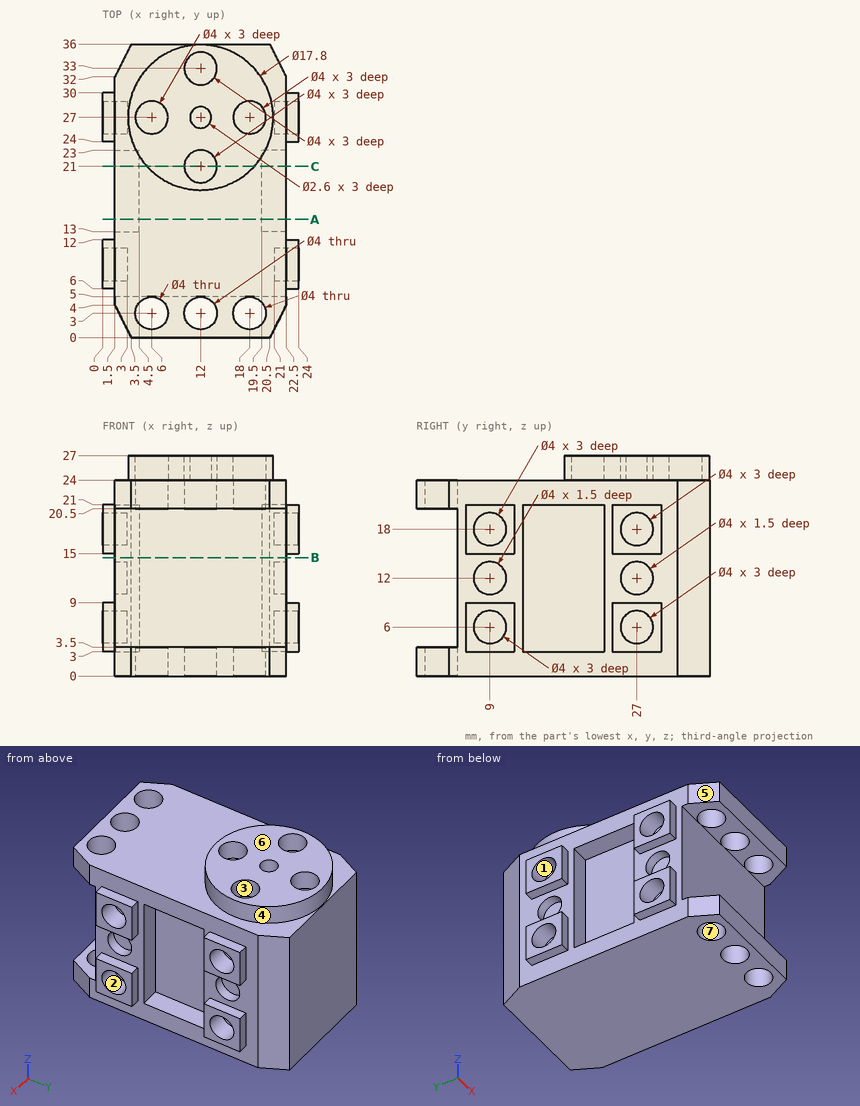
Answer from the drawing. Dimensions are ordinates in mm from the lowest x, y and z of the part. A direction names the side the tool comes from. Give positions to 0.01 mm unless a question says otherwise; leave off trailing zeros. Write each loop counter-clockwise with the first axis right and the second up, starting at its lowest first coordinate (ties: lowest second). Pieces come first, ordered by that corner, then holes.
1) Find the intervals of material crossed by L1, parallel to Y at x = 1.3, z = 6; L2, parallel to Y at x = 12, z = 2.8; L3, parallel to Y at x = 4, z = 4.75, in increasing order.
2) Section A-A (y = 14.5) is taken. Write down the section's boundary in (x, z), and give its area (3 significant figures).
3) Given P1, Ø2.5, axis at x = 6, y = 3, coming from the +Z side; P2, Ø1.2, axis at y = 27.5, z = 12, coming from the -X side; P3, Ø1.2, axis at x = 0.5, y = 8, coming from the +Z side; P4, Ø1, axis at y = 14.5, z = 21, coming from the -X side, each flat-ended and moving along its own axis, determine where each tip first touches the part or whether it passes through.
4) Section C-C (y = 21) is taken. Write down the section's boundary in (x, z).
5) For a pull along Y with two mould halves and no side action, classify the marked faces 4, 5, 6 and 7 as pulls with the +Y half, pulls with the -Y half, needs draft (parallel to the pull), parting line crosses it, or undercut.
6) A tool of negligible diameter and unlimited length cuts with its end or side. For the marked faces 1, 2 and 3, from which of +Z, -Z, +X, -X, +Y, -Y can it reach the whole face along a straight path? Write none if from no direction.
7) Section B-B (z = 14.5) is taken. Write down the section's boundary in (x, y), and give its area (3 significant figures).
Response:
1. L1: y = 6 to 7, 11 to 12, 24 to 25, 29 to 30
1. L2: y = 0 to 1, 5 to 36
1. L3: y = 5 to 13, 23 to 36
2. outline: (1.5, 0) - (22.5, 0) - (22.5, 3) - (19.5, 3) - (19.5, 21) - (22.5, 21) - (22.5, 24) - (1.5, 24) - (1.5, 21) - (4.5, 21) - (4.5, 3) - (1.5, 3) - close
2. area: 396 mm2
3. P1: passes through
3. P2: stops at x = 3
3. P3: stops at z = 21
3. P4: stops at x = 1.5
4. outline: (1.5, 0) - (22.5, 0) - (22.5, 3) - (19.5, 3) - (19.5, 21) - (22.5, 21) - (22.5, 24) - (18.57, 24) - (18.57, 27) - (14, 27) - (14, 24) - (10, 24) - (10, 27) - (5.43, 27) - (5.43, 24) - (1.5, 24) - (1.5, 21) - (4.5, 21) - (4.5, 3) - (1.5, 3) - close
5. face 4: parting line crosses it
5. face 5: pulls with the -Y half
5. face 6: needs draft
5. face 7: undercut
6. face 1: -X
6. face 2: +X
6. face 3: +Z
7. outline: (1.5, 5) - (22.5, 5) - (22.5, 13) - (19.5, 13) - (19.5, 23) - (22.5, 23) - (22.5, 32) - (20.5, 36) - (3.5, 36) - (1.5, 32) - (1.5, 23) - (4.5, 23) - (4.5, 13) - (1.5, 13) - close
7. area: 583 mm2
